Model file for the job. Use its own axes, mm. Face numbers are marked on the shaded views. A direction names the side the tool comes from. Give positions to 0.01 mm unless a question says otherwise; leave off trailing zeros. Write each loop counter-clockwise with the first axis right and the second up, starting at its lowest first coordinate (ties: lowest second). Pieces come first, ordered by that corner, then holes. Notation, with made-up numbers: M 86.25,-13.75 L 105.25,-13.75 A17 cw 105.25,10.25 Z; hole C -9,-24 d1. An arc over 180 degrees is marked long. Answer as a JSON object with one key per item and string values. Group by question number.
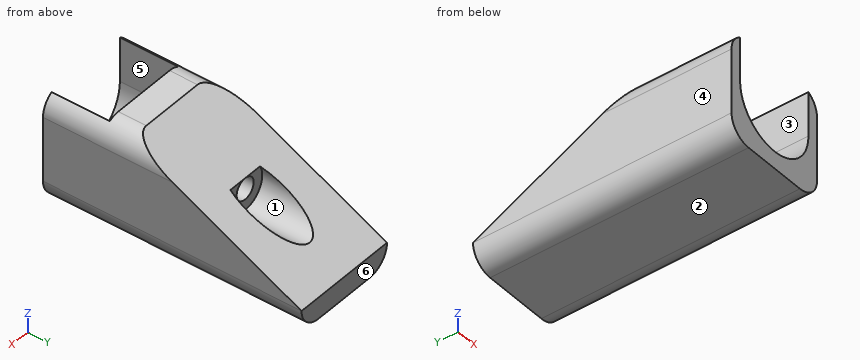
```python
from build123d import *

# Parameters (mm, degrees)
F0_W        = 25
F0_H        = 60
F1_DEPTH    = 25
F2_R        = 5
F4_DEPTH    = 13.5
F5_DEPTH    = 13.5
F6_T1_DEPTH = 222.1863099029
F7_R        = 2.5
F8_DEPTH    = 55
F10_START   = -23.5
F9_R        = 5
F10_DEPTH   = 23


# Not quite as in the source:
# - a fillet or chamfer that OpenCascade refuses, or shapes differently, is made with other operations: its cross-section is extruded or revolved along the edge and cut away or added
# - ends of sketch curves that miss each other by under 0.0002 mm in the source are joined


with BuildPart() as f1:
    # F0 (on Top) → F1 (new body)
    with BuildSketch(Plane.XY):
        Rectangle(F0_W, F0_H)
    extrude(amount=F1_DEPTH)

    # F2
    f2_edges = [f1.edges().sort_by_distance(p)[0] for p in [
        (12.5, 0, 25),
        (12.5, 0, 0),
        (-12.5, 0, 0),
        (-12.5, 0, 25),
    ]]
    fillet(f2_edges, radius=F2_R)

    # F3 (on face) → F4 (cut)
    with BuildSketch(Plane.XZ.offset(30)):
        with BuildLine():
            Line((-10, 13.9999993678), (10, 13.9999993678))
            ThreePointArc((10, 13.9999993678), (-3.161e-07, 24), (-10, 13.9999993678))
        make_face()
        with BuildLine():
            ThreePointArc((-10, 13.9999993678), (3.161e-07, 4), (10, 14))
            Line((10, 14), (-10, 13.9999993678))
        make_face()
    extrude(amount=-F4_DEPTH, mode=Mode.SUBTRACT)

    # F3 (on face) → F5 (cut)
    with BuildSketch(Plane.XZ.offset(30)):
        with BuildLine():
            ThreePointArc((-10, 13.9999993678), (-3.161e-07, 24), (10, 14))
            Line((10, 14), (10, 24.3301270189))
            ThreePointArc((10, 24.3301270189), (8.7940952255, 24.8296291314), (7.5, 25))
            Line((7.5, 25), (-7.5, 25))
            ThreePointArc((-7.5, 25), (-8.7940952255, 24.8296291314), (-10, 24.3301270189))
            Line((-10, 24.3301270189), (-10, 13.9999993678))
        make_face()
    extrude(amount=-F5_DEPTH, mode=Mode.SUBTRACT)

    # F6: chamfer of 40 x 20 on 1 edges, made by hand

    # F6_s2 → F6_t1 (cut)
    with BuildSketch(Plane.YZ.offset(-111.0931549515)):
        Polygon((30, 5), (-10, 25), (30, 25), align=None)
    extrude(amount=F6_T1_DEPTH, mode=Mode.SUBTRACT)

    # F7 (on face) → F8 (cut)
    with BuildSketch(Plane.XZ.offset(16.5)):
        with Locations((0, 14)):
            Circle(F7_R)
    extrude(amount=-F8_DEPTH, mode=Mode.SUBTRACT)

    # F9 (on face) → F10 (cut)
    with BuildSketch(Plane.XZ.offset(16.5).offset(F10_START)):
        with Locations((0, 14)):
            Circle(F9_R)
    extrude(amount=-F10_DEPTH, mode=Mode.SUBTRACT)


solid = f1.part
```
Q1. Slice it at A-A, the plane y = 4.5. Write the cut outline in (x, z).
Q2. Slice it at C-C, the plane z = 5.75. Write the cut outline in (x, y), then the cut area to 3 significant figures.
Q3. Slice it at D-D, the plane y = 16. Write the cut outline in (x, z).
Q4. Wall check: L1, parallel to X at y = 10.5, z = 14; L2, parallel to X at y = -17.5, z = 17.25; L3, parallel to Z at x = 6.5, y = 20. Give the ranges that are in metal, low to high.
Q5. 3-axis set-ups, long thin cutter, end or side, ignore diameter. For the marked faces 5 and 6: which of +Z, -Z, +X, -X, +Y, -Y reach the whole face in a straight line?
Q6. Two-plate mould, pull along X, no slides. Class the marked faces 1, 2, 3 and 4: +X half, -X half, draft (parallel to the pull), parting line (faces both ways), or undercut.
Q7. Slice it at B-B, the plane x = -6.5. Write the cut outline in (y, z).
Q8. Drop flat-ended pins along their axis: P1, Ø6, axis at x = 0, z = 14, coming from the +Y side; P2, Ø3, axis at x = 0, y = -23, coming from the +Z side; P3, Ø1, axis at x = -4.5, z = 9.5, coming from the +Y side. Give the stop position or say it passes through.
Solved:
{
 "1": {"outline": "M -12.5,5 A5 ccw -7.5,0 L 7.5,0 A5 ccw 12.5,5 L 12.5,17.75 L -12.5,17.75 Z; hole C 0,14 d5"},
 "2": {"outline": "M -12.5,-30 L -5.65,-30 L -5.65,-16.5 L 5.65,-16.5 L 5.65,-30 L 12.5,-30 L 12.5,28.5 L -12.5,28.5 Z", "area": "1,310 mm²"},
 "3": {"outline": "M -12.5,5 A5 ccw -7.5,0 L 7.5,0 A5 ccw 12.5,5 L 12.5,12 L 4.58,12 A5 cw -4.58,12 L -12.5,12 Z"},
 "4": {"L1": "x = -12.5 to -5, 5 to 12.5", "L2": "x = -12.5 to -10, 10 to 12.5", "L3": "z = 0 to 10"},
 "5": {"face 5": "+Z, -Y", "face 6": "+Z, -Z, +X, -X, +Y"},
 "6": {"face 1": "undercut", "face 2": "draft", "face 3": "undercut", "face 4": "-X half"},
 "7": {"outline": "M -30,0 L 30,0 L 30,5 L -10,25 L -16.5,25 L -16.5,6.4 L -30,6.4 Z"},
 "8": {"P1": "stops at y = 7", "P2": "stops at z = 4.11", "P3": "stops at y = 22"}
}
